Verification items for this drawing (mm, ordinates from the low corner). A direction names the side the tool comes from. Coordinates: 2 decimals unless noted, no trailing zeros. Use CSV: the item, a comma, the result in double quotes.
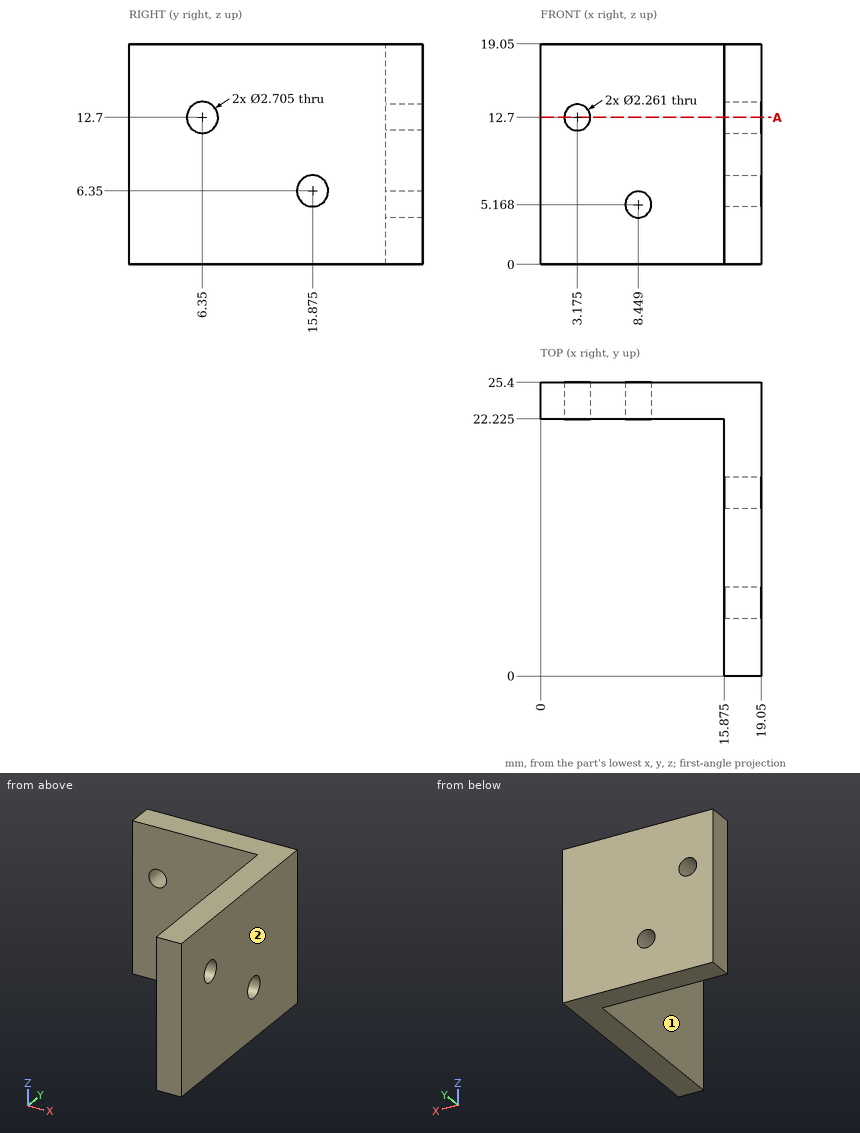
1. Set-up check for the marked faces 1 and 2: record each of +Z, -Z, +X, -X, +Y, -Y from which the full face is reachable in a straight line by a thin tool's end or side.
The answers:
face 1,"+Z, -Z, -X, -Y"
face 2,"+Z, -Z, +X, +Y, -Y"
2. Thickness scan on line 1 (Y direction, x = 7.5, z = 10) (1 decimal). Record the ranges inside material, lowest first. Write a range as [from, to].
The answers:
line 1,"[22.2, 25.4]"
3. Gauge pin test, flat ends, axial feed: P1, Ø2.5, axis at x = 3.175, z = 12.7, coming from the -Y side (3 decimals); P2, Ø3, axis at x = 16, y = 12.5, coming from the -Z side. Record the tip position at first contact, or that the pin passes through.
The answers:
P1,"y = 22.225"
P2,"z = 0"
4. Section check A-A, the plane z = 12.7. Count the separate pieces of the cut face and the enclosed holes in it, plus the area to 3 significant figures.
The answers:
separate pieces,"3"
enclosed holes,"0"
area,"115 mm^2"
